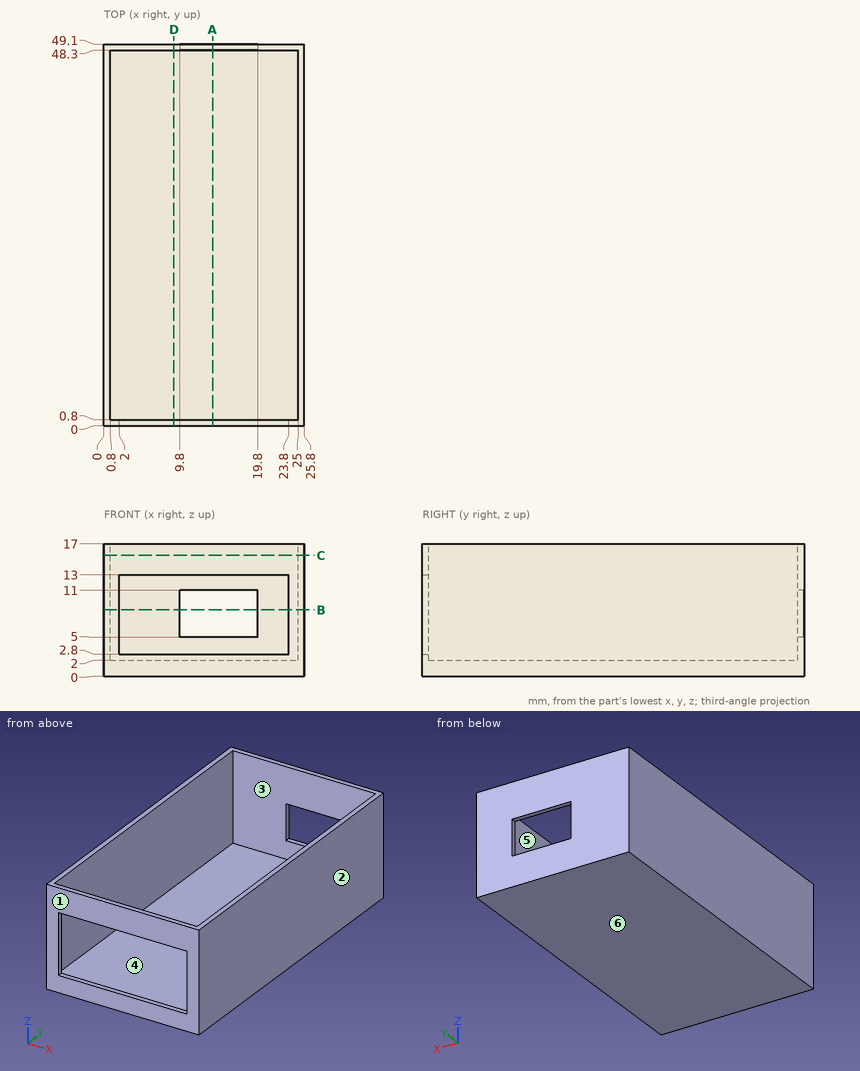
Input: dimensioned drawing with shaded views. Units: mm. Origin: part minimum x, y, z. A direction names the side the tool comes from. Round coordinates to 2 decimals unless told otherwise and drop trailing zeros. Loops run counter-clockwise (first coordinate to the right, second up) from the corner with the lowest first, then second, coordinate; pieces in that order, holes last. Notation, with made-up numbers: (67.25, 17) -> (106.25, 17) arc R32 ccw to (106.25, 52) -> close; hole circle Ø10 at (72.25, -29). An arc over 180 degrees is marked (long way). Use one line per item in the form item = value. Start each with the question number.
1) Section B-B on z = 8.5. Output: boundary loops of the cut face in (x, y), then the cut area to 3 significant figures.
2) First-contact query: P1, Ø4, axis at x = 7.5, y = 36.5, coming from the +Z side. Flat tip, straight axial feed; report the tip coordinate or a pass-through.
3) Line query: L1, parallel to X at y = 29, z = 7.75; L2, parallel to Y at x = 11.5, z = 15.5; L3, parallel to Z at x = 10.25, y = 3.5. Output: solid intervals per line, ascending.
4) Section D-D on x = 9. Output: boundary loops of the cut face in (y, z).
5) Access query for the marked faces 5 and 6. Directions: +Z, -Z, +X, -X, +Y, -Y. A direction counts if a zero-diameter tool reaches every point of the face in a straight line with its end or side. Return the directions, or none.
6) Section C-C on z = 15.5. Output: boundary loops of the cut face in (x, y).
7) Draft query along Y for the marked faces 1, 2, 3 and 4. Return one class per face: released by +Y, released by -Y, zero draft, split by the parting line, or undercut.
8) Section A-A on x = 14. Output: boundary loops of the cut face in (y, z).
Response:
q1.outline = (0, 0) -> (2, 0) -> (2, 0.8) -> (0.8, 0.8) -> (0.8, 48.3) -> (9.8, 48.3) -> (9.8, 49.1) -> (0, 49.1) -> close; (19.8, 48.3) -> (25, 48.3) -> (25, 0.8) -> (23.8, 0.8) -> (23.8, 0) -> (25.8, 0) -> (25.8, 49.1) -> (19.8, 49.1) -> close
q1.area = 91.8 mm^2
q2.P1 = 2
q3.L1 = 0 to 0.8, 25 to 25.8
q3.L2 = 0 to 0.8, 48.3 to 49.1
q3.L3 = 0 to 2
q4.outline = (0, 0) -> (49.1, 0) -> (49.1, 17) -> (48.3, 17) -> (48.3, 2) -> (0.8, 2) -> (0.8, 2.8) -> (0, 2.8) -> close; (0, 13) -> (0.8, 13) -> (0.8, 17) -> (0, 17) -> close
q5.face_5 = +Z
q5.face_6 = -Z, +X, -X, +Y, -Y
q6.outline = (0, 0) -> (25.8, 0) -> (25.8, 49.1) -> (0, 49.1) -> close; hole (0.8, 0.8) -> (25, 0.8) -> (25, 48.3) -> (0.8, 48.3) -> close
q7.face_1 = released by -Y
q7.face_2 = zero draft
q7.face_3 = undercut
q7.face_4 = undercut
q8.outline = (0, 0) -> (49.1, 0) -> (49.1, 5) -> (48.3, 5) -> (48.3, 2) -> (0.8, 2) -> (0.8, 2.8) -> (0, 2.8) -> close; (0, 13) -> (0.8, 13) -> (0.8, 17) -> (0, 17) -> close; (48.3, 11) -> (49.1, 11) -> (49.1, 17) -> (48.3, 17) -> close
